Here's how the part is built. I have some questions about the finished solid (model axes, mm). A direction names the side the tool comes from. Round coordinates to 2 decimals unless told otherwise and drop trailing zeros. Write each loop counter-clockwise with the first axis right and the second up, starting at its lowest first coordinate (ties: lowest second). Pieces come first, ordered by that corner, then holes. Notation, with made-up numbers: M 57,27 L 115,27 A31 ccw 115,57 Z; hole C -16.75,57 d6. An arc over 180 degrees is marked long. Use one line per item in the form item = value. Start each with the question number.
Q1. We'd pull the mould along Z, two halves only. Please class faces 1 (the face through (-94.721, -69.977, 1.283)), 2 (the face through (-62.186, 14.79, 105.547)), 3 (the face through (72.48, -50.07, -90.93)): +Z half, -Z half, draft (parallel to the pull), parting line (faces both ways), or undercut.
Q2. I need wall thicknesses on line 1 along X through (y, z) = (-58.75, 0); line 2 along X through (y, z) = (11, -1); line 3 along Y through (x, z) = (43, 4). Which ranges of each line are inside material? Lowest first, please. Write a range as from..to.
Q3. I'm going to push flat-ended pins straight in: pin 1 Ø3 at (y, z) = (2.5, 34.5) entering from +X; pin 2 Ø1.5 at (y, z) = (-17.5, -32.5) entering from -X; pin 3 Ø10 at (y, z) = (-19, 81) entering from +X. Where does each tip first touch, or does it pass through?
Q4. I want a section at B-B on z = 64.95. State how many separate pieces and enclosed holes the cut face has, and give its area (3 significant figures).
Q5. I want a section at A-A on y = 8.5. List the corners of the cut face in (x, z) for me, and give its area (3 significant figures).
Q6. For faces 4 (the face through (37.977, -74.37, 64.677)), 5 (the face through (52.034, 22.605, -88.314)), 6 (the face through (-11, -45, 0)), 7 (the face through (42.508, -50.066, 108.234)), which set-ups out of +Z, -Z, +X, -X, +Y, -Y let a thin tool reach every point of the face, with its end or its side?
```python
from build123d import *

# Parameters (mm, degrees)
BOSS_EXTRUDE2_DEPTH = 30
CUT_EXTRUDE1_DEPTH  = 15
BOSS_EXTRUDE4_DEPTH = 90
SKETCH7_R           = 10
CUT_EXTRUDE2_DEPTH  = 120
SKETCH8_R           = 25
CUT_EXTRUDE3_DEPTH  = 45
SKETCH9_R           = 40
CUT_EXTRUDE4_DEPTH  = 20
SKETCH10_R          = 6
CUT_EXTRUDE5_DEPTH  = 120
BOSS_EXTRUDE8_DEPTH = 40
SKETCH15_R          = 14
CUT_EXTRUDE7_DEPTH  = 40
SKETCH17_R          = 25
CUT_EXTRUDE8_DEPTH  = 15
CIRPATTERN1_COUNT   = 6


with BuildPart() as part:
    # Sketch3 → Boss-Extrude2 (new body)
    with BuildSketch(Plane(origin=(0, 0, 0), x_dir=(1, 0, 0), z_dir=(0, 1, 0))):
        Polygon((122.447087289, -70.816976409), (122.552844234, 70.633800007), (0.105756945, 141.450776416), (-122.447087289, 70.816976409), (-122.552844234, -70.633800007), (-0.105756945, -141.450776416), align=None)
    extrude(amount=BOSS_EXTRUDE2_DEPTH)

    # Sketch4 → Cut-Extrude1 (cut)
    with BuildSketch(Plane(origin=(0, 30, 0), x_dir=(1, 0, 0), z_dir=(0, 1, 0))):
        Polygon((102.455726099, -59.255021077), (102.544216604, 59.101751026), (0.088490505, 118.356772104), (-102.455726099, 59.255021077), (-102.544216604, -59.101751026), (-0.088490505, -118.356772104), align=None)
    extrude(amount=-CUT_EXTRUDE1_DEPTH, mode=Mode.SUBTRACT)

    # Sketch5 → Boss-Extrude4 (add)
    with BuildSketch(Plane.XZ):
        Polygon((75.032353613, -43.245183678), (74.967604463, 43.357332496), (-0.06474915, 86.602516173), (-75.032353613, 43.245183678), (-74.967604463, -43.357332496), (0.06474915, -86.602516173), align=None)
    extrude(amount=BOSS_EXTRUDE4_DEPTH)

    # Sketch7 → Cut-Extrude2 (cut)
    with BuildSketch(Plane.XZ.offset(90)):
        with Locations(Location((0, 0, 0), (0, 0, 270))):
            Circle(SKETCH7_R)
    extrude(amount=-CUT_EXTRUDE2_DEPTH, mode=Mode.SUBTRACT)

    # Sketch8 → Cut-Extrude3 (cut)
    with BuildSketch(Plane.XZ.offset(90)):
        with Locations(Location((0, 0, 0), (0, 0, 270))):
            Circle(SKETCH8_R)
    extrude(amount=-CUT_EXTRUDE3_DEPTH, mode=Mode.SUBTRACT)

    # Sketch9 → Cut-Extrude4 (cut)
    with BuildSketch(Plane.XZ.offset(90)):
        with Locations(Location((0, 0, 0), (0, 0, 270))):
            Circle(SKETCH9_R)
    extrude(amount=-CUT_EXTRUDE4_DEPTH, mode=Mode.SUBTRACT)

    # Sketch10 → Cut-Extrude5 (cut)
    with BuildSketch(Plane.XZ.offset(90)):
        with Locations(Location((0, 64.95, 0), (0, 0, 270))):
            Circle(SKETCH10_R)
        with Locations(Location((64.95, 0, 0), (0, 0, 270))):
            Circle(SKETCH10_R)
        with Locations(Location((0, -64.95, 0), (0, 0, 270))):
            Circle(SKETCH10_R)
        with Locations(Location((-64.95, 0, 0), (0, 0, 270))):
            Circle(SKETCH10_R)
    extrude(amount=-CUT_EXTRUDE5_DEPTH, mode=Mode.SUBTRACT)

    # Sketch12 → Boss-Extrude8 (add)
    with BuildSketch(Plane(origin=(74.999979038, 0, 0.056074409), x_dir=(0.0007476587847964174, 0, -0.9999997205031317), z_dir=(0.9999997205031318, 0, 0.0007476587847964174))):
        with BuildLine():
            Line((-26.457513111, 0), (26.457513111, 0))
            ThreePointArc((26.457513111, 0), (0, -70), (-26.457513111, 0))
        make_face()
    boss_extrude8 = extrude(amount=BOSS_EXTRUDE8_DEPTH)

    # Sketch15 → Cut-Extrude7 (cut)
    with BuildSketch(Plane(origin=(114.999967858, 0, 0.08598076), x_dir=(0.0007476587847964175, 0, -0.9999997205031317), z_dir=(0.9999997205031318, 0, 0.0007476587847964175))):
        with Locations((0, -30)):
            Circle(SKETCH15_R)
    cut_extrude7 = extrude(amount=-CUT_EXTRUDE7_DEPTH, mode=Mode.SUBTRACT)

    # Sketch17 → Cut-Extrude8 (cut)
    with BuildSketch(Plane(origin=(114.999967858, 0, 0.08598076), x_dir=(0.0007476587847964175, 0, -0.9999997205031317), z_dir=(0.9999997205031318, 0, 0.0007476587847964175))):
        with Locations((0, -30)):
            Circle(SKETCH17_R)
    cut_extrude8 = extrude(amount=-CUT_EXTRUDE8_DEPTH, mode=Mode.SUBTRACT)

    # CirPattern1: Boss-Extrude8, Cut-Extrude7, Cut-Extrude8 ×6 about axis
    cirpattern1_axis = Axis((0, 0, 0), (0, 1, 0))
    add([boss_extrude8.rotate(cirpattern1_axis, i * 360 / CIRPATTERN1_COUNT) for i in range(1, CIRPATTERN1_COUNT)])
    add([cut_extrude7.rotate(cirpattern1_axis, i * 360 / CIRPATTERN1_COUNT) for i in range(1, CIRPATTERN1_COUNT)], mode=Mode.SUBTRACT)
    add([cut_extrude8.rotate(cirpattern1_axis, i * 360 / CIRPATTERN1_COUNT) for i in range(1, CIRPATTERN1_COUNT)], mode=Mode.SUBTRACT)


solid = part.part
```
Reported:
q1.face_1 = undercut
q1.face_2 = +Z half
q1.face_3 = -Z half
q2.line_1 = -115..-70.95, -58.95..-25, 25..58.95, 70.95..115
q2.line_2 = -122.5..-70.87, -59.03..-9.95, 9.95..59.03, 70.87..122.5
q2.line_3 = -90..15
q3.pin_1 = 122.48
q3.pin_2 = -114.98
q3.pin_3 = 91.67
q4.separate_pieces = 2
q4.enclosed_holes = 2
q4.area = 14,700 mm^2
q5.outline = M -122.55,70.63 L -122.45,-70.82 L 0.11,-141.45 L 122.55,-70.63 L 122.45,70.82 L -0.11,141.45 Z; hole C -64.95,0 d12; hole C 0,0 d20; hole C 0,-64.95 d12; hole C 0,64.95 d12; hole C 64.95,0 d12
q5.area = 51,200 mm^2
q6.face_4 = none
q6.face_5 = +Y
q6.face_6 = -Y
q6.face_7 = +Z, +X, -Y
